Input: part model. Units: mm. Frame: model coordinates. Face numbers are marked on the shaded views. A direction names the side the tool comes from. Round coordinates to 2 decimals unless told otherwise and drop trailing zeros. Write each loop counter-clockwise with the first axis right and the second up, starting at its lowest first coordinate (ties: lowest second). Pieces come first, ordered by that corner, then holes. Notation, with made-up numbers: M 47.25,3 L 82.25,3 A33 ccw 82.25,35 Z; hole C 66,-24.5 d2. An arc over 180 degrees is marked long. Answer as CSV lines item,"result". Start each with the question number.
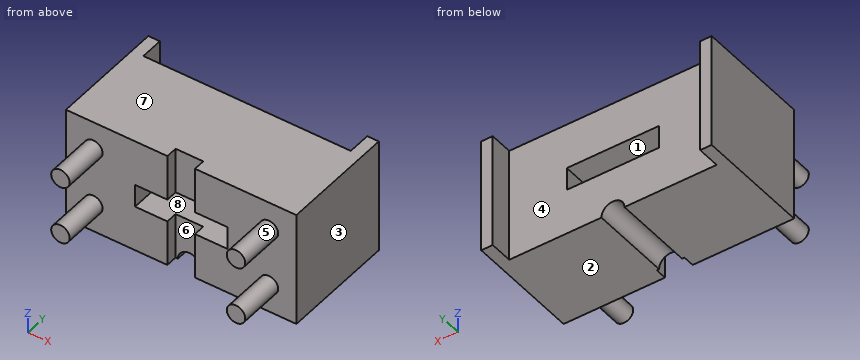
```python
from build123d import *

# Parameters (mm, degrees)
SKETCH_1_W          = 10
SKETCH_1_H          = 5
EXTRUDE_1_DEPTH     = 5
CUT_EXTRUDE_1_REACH = 14.247
SKETCH_2_R          = 0.5
CUT_EXTRUDE_2_REACH = 14.247
SKETCH_4_W          = 4.5
SKETCH_4_H          = 1
SKETCH_4_W_2        = 0.6
SKETCH_4_H_2        = 0.5
CUT_EXTRUDE_3_REACH = 13.874
SKETCH_5_W          = 4
SKETCH_5_H          = 1
SKETCH_6_R          = 0.4
EXTRUDE_2_DEPTH     = 2


with BuildPart() as part:
    # 草图1 → 凸台-拉伸1 (new body)
    with BuildSketch(Plane(origin=(0, 0, 0), x_dir=(1, 0, 0), z_dir=(0, 1, 0))):
        with Locations((5, 2.5)):
            Rectangle(SKETCH_1_W, SKETCH_1_H)
    extrude(amount=EXTRUDE_1_DEPTH)

    # 草图2 → 切除-拉伸1 (cut, up to next)
    with BuildSketch(Plane(origin=(0, 5, 0), x_dir=(-1, 0, 0), z_dir=(0, 1, 0)), mode=Mode.PRIVATE) as cut_extrude_1_sk1:
        with Locations((-5, -5)):
            Circle(SKETCH_2_R)
    cut_extrude_1_tool1 = extrude(cut_extrude_1_sk1.sketch, amount=-CUT_EXTRUDE_1_REACH, mode=Mode.PRIVATE) & part.part
    add(cut_extrude_1_tool1.solids().sort_by_distance((5, 5, -5))[0], mode=Mode.SUBTRACT)

    # 草图4 → 切除-拉伸2 (cut, up to next)
    with BuildSketch(Plane.XY, mode=Mode.PRIVATE) as cut_extrude_2_sk1:
        with Locations((2.75, 4.5)):
            Rectangle(SKETCH_4_W, SKETCH_4_H)
    cut_extrude_2_tool1 = extrude(cut_extrude_2_sk1.sketch, amount=-CUT_EXTRUDE_2_REACH, mode=Mode.PRIVATE) & part.part
    # 草图4 → 切除-拉伸2 (cut, up to next)
    with BuildSketch(Plane.XY, mode=Mode.PRIVATE) as cut_extrude_2_sk2:
        with Locations((7.25, 4.5)):
            Rectangle(SKETCH_4_W, SKETCH_4_H)
    cut_extrude_2_tool2 = extrude(cut_extrude_2_sk2.sketch, amount=-CUT_EXTRUDE_2_REACH, mode=Mode.PRIVATE) & part.part
    # 草图4 → 切除-拉伸2 (cut, up to next)
    with BuildSketch(Plane.XY, mode=Mode.PRIVATE) as cut_extrude_2_sk3:
        with Locations((4.7, 0.25)):
            Rectangle(SKETCH_4_W_2, SKETCH_4_H_2)
    cut_extrude_2_tool3 = extrude(cut_extrude_2_sk3.sketch, amount=-CUT_EXTRUDE_2_REACH, mode=Mode.PRIVATE) & part.part
    # 草图4 → 切除-拉伸2 (cut, up to next)
    with BuildSketch(Plane.XY, mode=Mode.PRIVATE) as cut_extrude_2_sk4:
        with Locations((5.3, 0.25)):
            Rectangle(SKETCH_4_W_2, SKETCH_4_H_2)
    cut_extrude_2_tool4 = extrude(cut_extrude_2_sk4.sketch, amount=-CUT_EXTRUDE_2_REACH, mode=Mode.PRIVATE) & part.part
    add(cut_extrude_2_tool1.solids().sort_by_distance((2.75, 4.5, 0))[0], mode=Mode.SUBTRACT)
    add(cut_extrude_2_tool2.solids().sort_by_distance((7.25, 4.5, 0))[0], mode=Mode.SUBTRACT)
    add(cut_extrude_2_tool3.solids().sort_by_distance((4.7, 0.25, 0))[0], mode=Mode.SUBTRACT)
    add(cut_extrude_2_tool4.solids().sort_by_distance((5.3, 0.25, 0))[0], mode=Mode.SUBTRACT)

    # 草图5 → 切除-拉伸3 (cut, up to next)
    with BuildSketch(Plane(origin=(0, 4, 0), x_dir=(1, 0, 0), z_dir=(0, 1, 0)), mode=Mode.PRIVATE) as cut_extrude_3_sk1:
        with Locations((5, 2.5)):
            Rectangle(SKETCH_5_W, SKETCH_5_H)
    cut_extrude_3_tool1 = extrude(cut_extrude_3_sk1.sketch, amount=-CUT_EXTRUDE_3_REACH, mode=Mode.PRIVATE) & part.part
    add(cut_extrude_3_tool1.solids().sort_by_distance((5, 4, -2.5))[0], mode=Mode.SUBTRACT)

    # 草图6 → 凸台-拉伸2 (add)
    with BuildSketch(Plane.XZ):
        with Locations(Location((1.19, -1.23, 0), (0, 0, 90))):
            Circle(SKETCH_6_R)
        with Locations(Location((1.19, -3.77, 0), (0, 0, 90))):
            Circle(SKETCH_6_R)
        with Locations(Location((8.81, -3.77, 0), (0, 0, 90))):
            Circle(SKETCH_6_R)
        with Locations(Location((8.81, -1.23, 0), (0, 0, 90))):
            Circle(SKETCH_6_R)
    extrude(amount=EXTRUDE_2_DEPTH)


solid = part.part
```
Item 1: Cut plane B-B, the plane y = 0.75. Return loops of the section in (x, z), plus the area to 3 significant figures.
Item 2: Cut plane D-D, the plane x = 8.81. Return loops of the section in (y, z).
Item 3: Access query for the marked faces 4, 5, 6, 7 and 8. Directions: +Z, -Z, +X, -X, +Y, -Y. A direction counts if a zero-diameter tool reaches every point of the face in a straight line with its end or side. Return the directions, or none.
Item 4: Line query: line 1 (Z direction, x = 5, y = 2); line 2 (Y direction, x = 1.75, z = -1.8); line 3 (X direction, y = 0.25, z = -0.9). Output: solid intervals per line, ascending. Write a range as [from, to].
Item 5: Pin query (flat end, axial travel): pin 1 Ø3 at (x, y) = (5.5, 2.5) entering from +Z; pin 2 Ø2.5 at (x, z) = (5.5, -2.5) entering from +Y; pin 3 Ø0.6 at (x, z) = (5, -0.5) entering from -Y; pin 4 Ø1.3 at (x, z) = (5, -4) entering from -Y. Return the tip coordinate at first contact, or that it passes through.
Item 6: Cut plane A-A, the plane x = 5. Return loops of the section in (y, z).
Item 7: Cut plane C-C, the plane z = -1.23. Return loops of the section in (x, y), plus the area to 3 significant figures.
Item 8: Draft query along X for the marked faces 1, 2 and 3. Return one class per face: +X half, -X half, draft (parallel to the pull), parting line (faces both ways), or undercut.
Results list:
1,outline,"M 0,-5 L 4.5,-5 A0.5 cw 5.5,-5 L 10,-5 L 10,0 L 0,0 Z; hole M 3,-3 L 7,-3 L 7,-2 L 3,-2 Z"
1,area,"45.6 mm²"
2,outline,"M -2,-4.17 L 0,-4.17 L 0,-5 L 4,-5 L 4,0 L 0,0 L 0,-0.83 L -2,-0.83 L -2,-1.63 L 0,-1.63 L 0,-3.37 L -2,-3.37 Z"
3,face 4,"+Z, -Z, +Y"
3,face 5,"-Y"
3,face 6,"+Z, -Z, -Y"
3,face 7,"+Z, +X, -X, +Y, -Y"
3,face 8,"+Y, -Y"
4,line 1,"[-4.5, -3], [-2, 0]"
4,line 2,"[0, 4]"
4,line 3,"[0, 4.4], [5.6, 10]"
5,pin 1,"z = 0"
5,pin 2,"y = 4"
5,pin 3,"y = 0.5"
5,pin 4,"y = 0"
6,outline,"M 0.5,-4.5 L 4,-4.5 L 4,-3 L 0.5,-3 Z; M 0.5,-2 L 4,-2 L 4,0 L 0.5,0 Z"
7,outline,"M 0,0 L 0.79,0 L 0.79,-2 L 1.59,-2 L 1.59,0 L 4.4,0 L 4.4,0.5 L 5.6,0.5 L 5.6,0 L 8.41,0 L 8.41,-2 L 9.21,-2 L 9.21,0 L 10,0 L 10,5 L 9.5,5 L 9.5,4 L 0.5,4 L 0.5,5 L 0,5 Z"
7,area,"43.6 mm²"
8,face 1,"undercut"
8,face 2,"draft"
8,face 3,"+X half"
